```python
from build123d import *

# Parameters (mm, degrees)
SKETCH_5_R  = 43
SKETCH_6_R  = 43
SKETCH_3_R  = 32.8
SKETCH_4_R  = 41.75
SKETCH_2_R  = 30.775
SKETCH_1_R  = 30
SKETCH_11_R = 29
SKETCH_12_R = 29.775
SKETCH_13_R = 40
SKETCH_14_R = 31.8


with BuildPart() as part:
    # 草图5 → Loft 2 section 0
    with BuildSketch(Plane(origin=(0, 132.3, 0), x_dir=(1, 0, 0), z_dir=(0, 1, 0))):
        Circle(SKETCH_5_R)
    # 草图6 → Loft 2 section 1
    with BuildSketch(Plane(origin=(0, 135.8, 0), x_dir=(1, 0, 0), z_dir=(0, 1, 0))):
        Circle(SKETCH_6_R)
    loft()

    # 草图3 → 放样3 section 0
    with BuildSketch(Plane(origin=(0, 11, 0), x_dir=(1, 0, 0), z_dir=(0, 1, 0))):
        Circle(SKETCH_3_R)
    # 草图4 → 放样3 section 1
    with BuildSketch(Plane(origin=(0, 132.3, 0), x_dir=(1, 0, 0), z_dir=(0, 1, 0))):
        Circle(SKETCH_4_R)
    loft()

    # 草图2 → 放样4 section 0
    with BuildSketch(Plane(origin=(0, 11, 0), x_dir=(1, 0, 0), z_dir=(0, 1, 0))):
        Circle(SKETCH_2_R)
    # 草图1 → 放样4 section 1
    with BuildSketch(Plane(origin=(0, 0, 0), x_dir=(1, 0, 0), z_dir=(0, 1, 0))):
        Circle(SKETCH_1_R)
    loft()

    # 草图11 → 切除-放样1 section 0
    with BuildSketch(Plane(origin=(0, 0, 0), x_dir=(1, 0, 0), z_dir=(0, 1, 0))):
        Circle(SKETCH_11_R)
    # 草图12 → 切除-放样1 section 1
    with BuildSketch(Plane(origin=(0, 11, 0), x_dir=(1, 0, 0), z_dir=(0, 1, 0))):
        Circle(SKETCH_12_R)
    loft(mode=Mode.SUBTRACT)

    # 草图13 → Loft 2 2 section 0
    with BuildSketch(Plane(origin=(0, 135.8, 0), x_dir=(1, 0, 0), z_dir=(0, 1, 0))):
        Circle(SKETCH_13_R)
    # 草图14 → Loft 2 2 section 1
    with BuildSketch(Plane(origin=(0, 12, 0), x_dir=(1, 0, 0), z_dir=(0, 1, 0))):
        Circle(SKETCH_14_R)
    loft(mode=Mode.SUBTRACT)


solid = part.part
```
Geometry: final body of the model. Coordinates: model frame, mm. A direction names the side the tool comes from. Give positions to 0.01 mm unless a question says otherwise; leave off trailing zeros. Order: outer loops, then holes, each group sorted by start corner. A loop starts at its lowest first (then second) coordinate and runs counter-clockwise, first axis right, second up. Notation, with made-up numbers: (-32.5, -2.75) -> (11.5, -2.75) arc R37 cw to (11.5, 36.25) -> close; hole circle Ø11 at (59.25, -1). An arc over 180 degrees is marked (long way). Write each question's results on one line, items separated by ' | '. Start each with the question number.
1) First-contact query: pin 1 (4 mm diameter, centred on x = -9.5, z = -6, fed in from -Y); pin 2 (12 mm diameter, centred on y = 120, z = -3, fed in from -X); pin 3 (12 mm diameter, centred on x = 23.5, y = 17, fed in from +Z). Flat tips, straight axial feed; report the tip coordinate or a pass-through.
2) Section B-B (y = 101.5). Return loops of the section in (x, z).
3) Line query: line 1 (Y direction, x = 4.5, z = 7); line 2 (Z direction, x = -8.5, y = 129); line 3 (Z direction, x = 7, y = 15). Output: solid intervals per line, ascending. Write a range as from..to.
4) Section C-C (y = 22.5). Return loops of the section in (x, z).
5) Section A-A (x = 0). Return loops of the section in (y, z) (3 decimals).
6) Draft query along Z for faces 4 (the flat face through (-7, 132.3, -42)), 5 (the conical face through (-23.974, 2.979, 18.382)), 6 (the conical face through (-6.334, 3.133, 28.526)). Return one class per face: pulls with the +Z half, pulls with the -Z half, needs draft (parallel to the pull), parting line crosses it, or undercut.
7) Set-up query: faces 1 (the cylindrical face through (-5.598, 134.074, -42.634)), 2 (the flat face through (0, 12, 0)), 3 (the flat face through (-9.9, 11, -29.3)). Return all of +Z, -Z, +X, -X, +Y, -Y with unobstructed straight access to the full face (end or side cutting, diameter ignored); none if empty.
Calculated:
1) pin 1: y = 11 | pin 2: x = -41.25 | pin 3: z = 28.3
2) outline: circle Ø78.95 at (0, 0); hole circle Ø75.46 at (0, 0)
3) line 1: 11..12 | line 2: -40.63..-38.63, 38.63..40.63 | line 3: -32.35..-31.22, 31.22..32.35
4) outline: circle Ø67.3 at (0, 0); hole circle Ø64.99 at (0, 0)
5) outline: (0, -30) -> (11, -30.775) -> (11, -32.8) -> (132.3, -41.75) -> (132.3, -43) -> (135.8, -43) -> (135.8, -40) -> (12, -31.8) -> (12, 31.8) -> (135.8, 40) -> (135.8, 43) -> (132.3, 43) -> (132.3, 41.75) -> (11, 32.8) -> (11, 30.775) -> (0, 30) -> (0, 29) -> (11, 29.775) -> (11, -29.775) -> (0, -29) -> close
6) face 4: needs draft | face 5: parting line crosses it | face 6: undercut
7) face 1: +Y, -Y | face 2: +Y | face 3: -Y
